Geometry check sheet. Reference: the model listing, model coordinates, mm. Face numbers are marked on the shaded views. A direction names the side the tool comes from. Coordinates: 2 decimals unless noted, no trailing zeros. Write each loop counter-clockwise with the first axis right and the second up, starting at its lowest first coordinate (ties: lowest second). Pieces come first, ordered by that corner, then holes. Notation, with made-up numbers: M 9,-25.75 L 17,-25.75 A18 cw 17,-12.75 Z; hole C 26.25,16.25 d4. An arc over 180 degrees is marked long. Write each question's results on one line, items separated by ' | '.
Autodesk Inventor part; units mm, degrees
ref_plane "YZ Plane" through (0, 0, 0) normal (1, 0, 0) x (0, 1, 0)
ref_plane "XZ Plane" through (0, 0, 0) normal (0, 1, 0) x (-1, 0, 0)
ref_plane "XY Plane" through (0, 0, 0) normal (0, 0, 1) x (1, 0, 0)
ref_plane "Work Plane1" through (0, 0, 108.3756) normal (0, 0, 1) x (1, 0, 0)
sketch "Sketch1" plane through (0, 0, 108.3756) normal (0, 0, 1) x (1, 0, 0)
  line L0 (-71.3, 18) -> (-71.3, -18)
  line L1 (-71.3, -18) -> (-211.3, -18)
  line L2 (-211.3, -18) -> (-211.3, 18)
  line L3 (-211.3, 18) -> (-71.3, 18)
  line L4 (71.3003, -18) -> (71.3003, 18)
  line L5 (71.3003, 18) -> (211.3003, 18)
  line L6 (211.3003, 18) -> (211.3003, -18)
  line L7 (211.3003, -18) -> (71.3003, -18)
  line L8 (-241.3, 22) -> (241.3, 22)
  line L9 (-241.3, -22) -> (-241.3, 22)
  line L10 (241.3, -22) -> (-241.3, -22)
  line L11 (241.3, 22) -> (241.3, -22)
  circle A0 centre (-232.5, -15.875) radius 3.5
  circle A1 centre (-232.5, 15.875) radius 3.5
  circle A2 centre (232.5, -15.875) radius 3.5
  circle A3 centre (232.5, 15.875) radius 3.5
  line L12 (-219.3, 10) -> (-219.3, -10)
  line L13 (-63.3, 10) -> (-63.3, -10)
  arc A4 (-211.3, 18) -> (-219.3, 10) centre (-211.3, 10) ccw
  arc A5 (-219.3, -10) -> (-211.3, -18) centre (-211.3, -10) ccw
  arc A6 (-63.3, 10) -> (-71.3, 18) centre (-71.3, 10) ccw
  arc A7 (-71.3, -18) -> (-63.3, -10) centre (-71.3, -10) ccw
  line L14 (-211.3, 18) -> (-71.3, 18)
  line L15 (-71.3, -18) -> (-211.3, -18)
  circle A8 centre (-215.3, 0) radius 2
  circle A9 centre (-67.3, 0) radius 2
  point P0 (0, 0)
  point P1 (-63.3, 0)
  dimension "d0" = 8
  dimension "d1" = 8
  dimension "d5" = 4
  dimension "d6" = 4
  dimension "d7" = 18
  dimension "d9" = 4
  dimension "d106" = 18
extrude "Extrusion2" add sketch "Sketch1" along normal blind 2 contours A6 L13 A7 L0 | L0 L1 L2 L3 | L2 A5 L12 A4
ref_plane "Work Plane4" through (-211.3, -18, 108.3756) normal (0, -1, 0) x (1, 0, 0)
sketch "Sketch3" plane through (-211.3, -18, 108.3756) normal (0, -1, 0) x (1, 0, 0)
  line L0 (0, 2) -> (140, 2)
  line L1 (0, 2) -> (140, 2)
  line L2 (140, 2) -> (140, 102)
  line L3 (140, 102) -> (0, 102)
  line L4 (0, 102) -> (0, 2)
  point P0 (211.3, -108.3756)
  point P1 (140, 2)
  dimension "d14" = 100
  dimension "d15" = 0
extrude "Extrusion3" add sketch "Sketch3" against normal blind 2
ref_plane "Work Plane5" through (-71.3, -18, 210.3756) normal (1, 0, 0) x (0, 0, -1)
sketch "Sketch4" plane through (-71.3, -18, 210.3756) normal (1, 0, 0) x (0, 0, -1)
  line L0 (0, 2) -> (100, 2)
  line L1 (100, 2) -> (1, 2)
  line L2 (1, 2) -> (100, 36)
  line L3 (100, 36) -> (100, 2)
  point P0 (210.3756, 18)
  dimension "d19" = 99
extrude "Side" add sketch "Sketch4" against normal blind 2
ref_plane "Work Plane6" through (-211.3, -18, 110.3756) normal (-1, 0, 0) x (0, 0, 1)
sketch "Sketch5" plane through (-211.3, -18, 110.3756) normal (-1, 0, 0) x (0, 0, 1)
  line L0 (0, 2) -> (100, 2)
  line L1 (0, 2) -> (99, 2)
  line L2 (0, 36) -> (99, 2)
  line L3 (0, 36) -> (99, 2)
  line L4 (0, 36) -> (0, 2)
  point P0 (-110.3756, 18)
extrude "Extrusion5" add sketch "Sketch5" against normal blind 2
sketch "Sketch7" plane through (0, 0, 110.3756) normal (0, 0, 1) x (1, 0, 0)
  line L0 (-209.3, -16) -> (-73.3, -16)
  line L1 (-129.3, -16) -> (-204.3, -16)
  line L2 (-134.3, 18) -> (-209.3, 18)
  line L3 (-134.3, -18) -> (-134.3, 18)
  line L4 (-209.3, 18) -> (-209.3, -16)
  line L5 (-209.3, -18) -> (-134.3, -18)
  line L6 (-209.3, -18) -> (-134.3, -18)
  line L7 (-209.3, 18) -> (-134.3, 18)
  line L8 (-134.3, 18) -> (-134.3, -18)
  line L9 (-134.3, -18) -> (-209.3, -18)
  line L10 (-209.3, -18) -> (-209.3, 18)
  point P0 (0, 0)
  point P1 (-134.3, -16)
extrude "Extrusion7" cut sketch "Sketch7" against normal through all contours L4 L2 L3 L0
sketch "Sketch14" plane through (0, 0, 108.3756) normal (0, 0, -1) x (-1, 0, 0)
  line L0 (116.3, 1.1) -> (131.8, 1.1)
  line L1 (110.85, 3.1) -> (99.75, 3.1)
  line L2 (80.95, 3.1) -> (93.65, 3.1)
  line L3 (131.8, -12.2) -> (131.8, 0.9)
  line L4 (116.3, 0.9) -> (116.3, -12.2)
  line L5 (112.15, -1.76) -> (112.15, 2.24)
  line L6 (112.15, -10.26) -> (112.15, -6.26)
  line L7 (98.05, -6.56) -> (98.05, -9.96)
  line L8 (98.05, 1.94) -> (98.05, -1.46)
  line L9 (81.3, -12.4) -> (131.3, -12.4)
  line L10 (94.1, -5.96) -> (94.1, -9.76)
  line L11 (94.1, -2.3) -> (94.1, 1.5)
  line L12 (80.5, -2.3) -> (80.5, 1.5)
  line L13 (80.5, -5.96) -> (80.5, -9.76)
  line L14 (79.5, 4.1) -> (95.1, 4.1)
  line L15 (95.1, 4.1) -> (95.1, -13.4)
  line L16 (95.1, -13.4) -> (79.5, -13.4)
  line L17 (79.5, -13.4) -> (79.5, 4.1)
  line L18 (97.05, 4.1) -> (113.15, 4.1)
  line L19 (113.15, 4.1) -> (113.15, -13.4)
  line L20 (113.15, -13.4) -> (97.05, -13.4)
  line L21 (97.05, -13.4) -> (97.05, 4.1)
  line L22 (115.3, 2.1) -> (132.8, 2.1)
  line L23 (132.8, 2.1) -> (132.8, -13.4)
  line L24 (132.8, -13.4) -> (115.3, -13.4)
  line L25 (115.3, -13.4) -> (115.3, 2.1)
  point P0 (0, 0)
  dimension "d54" = 1
  dimension "d55" = 1
  dimension "d56" = 1
  dimension "d58" = 1
  dimension "d59" = 1
  dimension "d60" = 1
  dimension "d61" = 1
  dimension "d62" = 1
  dimension "d63" = 1
  dimension "d64" = 1
  dimension "d65" = 1
  dimension "d66" = 1
extrude "Extrusion12" cut sketch "Sketch14" against normal up to surface (2 mm away)
fillet "Fillet1" radius 1.5 2 edges at (-69.3, 0, 108.3756) (-217.3, 0, 108.3756)
sketch "Sketch19" plane through (0, 0, 108.3756) normal (0, 0, -1) x (-1, 0, 0)
  circle A0 centre (67.3, 0) radius 3.5
  line L0 (79.5, 4.1) -> (95.1, 4.1)
  line L1 (95.1, 4.1) -> (95.1, -13.4)
  line L2 (95.1, -13.4) -> (79.5, -13.4)
  line L3 (79.5, -13.4) -> (79.5, 4.1)
  line L4 (132.8, -13.4) -> (115.3, -13.4)
  line L5 (115.3, -13.4) -> (115.3, 2.1)
  line L6 (115.3, 2.1) -> (132.8, 2.1)
  line L7 (132.8, 2.1) -> (132.8, -13.4)
  line L8 (97.05, -13.4) -> (97.05, 4.1)
  line L9 (97.05, 4.1) -> (113.15, 4.1)
  line L10 (113.15, 4.1) -> (113.15, -13.4)
  line L11 (113.15, -13.4) -> (97.05, -13.4)
  line L12 (209.3, 18) -> (209.3, -16)
  line L13 (209.3, -16) -> (134.3, -16)
  line L14 (134.3, -16) -> (134.3, 18)
  line L15 (71.3, 18) -> (134.3, 18)
  arc A1 (71.3, 18) -> (63.3, 10) centre (71.3, 10) ccw
  line L16 (63.3, -10) -> (63.3, 10)
  arc A2 (63.3, -10) -> (71.3, -18) centre (71.3, -10) ccw
  line L17 (211.3, -18) -> (71.3, -18)
  arc A3 (211.3, -18) -> (219.3, -10) centre (211.3, -10) ccw
  line L18 (219.3, 10) -> (219.3, -10)
  arc A4 (219.3, 10) -> (211.3, 18) centre (211.3, 10) ccw
  line L19 (209.3, 18) -> (211.3, 18)
  circle A5 centre (215.3, 0) radius 3.5
  line L20 (71.3, 21) -> (211.3, 21)
  line L21 (63.3, 10) -> (63.3, 13)
  line L22 (63.3, -10) -> (63.3, -13)
  line L23 (219.3, 10) -> (219.3, 13)
  line L24 (219.3, -10) -> (219.3, -13)
  line L25 (71.3, -21) -> (211.3, -21)
  arc A6 (211.3, -21) -> (219.3, -13) centre (211.3, -13) ccw
  arc A7 (219.3, 13) -> (211.3, 21) centre (211.3, 13) ccw
  arc A8 (71.3, 21) -> (63.3, 13) centre (71.3, 13) ccw
  arc A9 (63.3, -13) -> (71.3, -21) centre (71.3, -13) ccw
  line L26 (209.3, 18) -> (134.3, 18)
  point P0 (0, 0)
  dimension "d108" = 3
  dimension "d109" = 3
  dimension "d110" = 3
  dimension "d111" = 3
  dimension "d112" = 3
  dimension "d114" = 3
extrude "Extrusion17" add sketch "Sketch19" against normal blind 2 contours L26 L15 A1 L21 A8 L20 A7 L23 A4 L19 | L24 A6 L25 A9 L22 A2 L17 A3
sketch "Sketch20" plane through (-71.3, -18, 210.3756) normal (1, 0, 0) x (0, 0, -1)
  line L0 (100, 36) -> (1, 2)
  line L1 (1, 2) -> (1, 17)
  line L2 (102, 36) -> (100, 36)
  line L3 (1, 17) -> (100, 36)
  point P0 (210.3756, 18)
  dimension "d117" = 15
extrude "Extrusion18" add sketch "Sketch20" against normal blind 2
sketch "Sketch21" plane through (-71.3, -18, 210.3756) normal (1, 0, 0) x (0, 0, -1)
  line L0 (1, 2) -> (100, 2)
  line L1 (100, 36) -> (1, 17)
  line L2 (16, 2) -> (51, 2)
  line L3 (51, 2) -> (51, 11)
  line L4 (45, 17) -> (22, 17)
  line L5 (16, 11) -> (16, 2)
  line L6 (1, 17) -> (1, 2)
  arc A0 (22, 17) -> (16, 11) centre (22, 11) ccw
  arc A1 (51, 11) -> (45, 17) centre (45, 11) ccw
  arc A2 (16, 7) -> (21, 2) centre (21, 7) ccw
  arc A3 (46, 2) -> (51, 7) centre (46, 7) ccw
  point P0 (210.3756, 18)
  point P1 (21, 2)
  point P2 (46, 2)
  dimension "d120" = 15
  dimension "d121" = 15
  dimension "d122" = 50
  dimension "d123" = 6
  dimension "d124" = 5
  dimension "d125" = 5
extrude "Extrusion19" cut sketch "Sketch21" against normal blind 2 contours A2 L5 A0 L4 A1 L3 A3 L0
sketch "Sketch24" plane through (-211.3, -16, 108.3756) normal (0, 1, 0) x (1, 0, 0)
  circle A0 centre (129.5, -25.5) radius 1.35
  circle A1 centre (80.5, -25.5) radius 1.35
  circle A2 centre (80.5, -83.5) radius 1.35
  circle A3 centre (129.5, -83.5) radius 1.35
  circle A4 centre (129.5, -83.5) radius 3.5
  circle A5 centre (80.5, -83.5) radius 3.5
  circle A6 centre (80.5, -25.5) radius 3.5
  circle A7 centre (129.5, -25.5) radius 3.5
  point P0 (211.3, 108.3756)
  dimension "d128" = 7
  dimension "d129" = 7
  dimension "d130" = 7
  dimension "d131" = 7
extrude "Extrusion20" add sketch "Sketch24" along normal blind 2 contours A0 | A1 | A2 | A3 | A4 | A5 | A6 | A7
sketch "Sketch25" plane through (-130.8, -14, 133.8756) normal (0, 1, 0) x (1, 0, 0)
  circle A0 centre (49, 0) radius 3.5
  circle A1 centre (49, -58) radius 3.5
  circle A2 centre (0, -58) radius 3.5
  circle A3 centre (0, 0) radius 3.5
  point P0 (130.8, 133.8756)
hole "Hole1" at (-81.8, -14, 133.8756) at (-130.8, -14, 133.8756) at (-130.8, -14, 191.8756) at (-81.8, -14, 191.8756) direction (0, -1, 0) diameter 2 end through all
properties part number "RPI_HOUSING2" material "Rubber, Silicone"
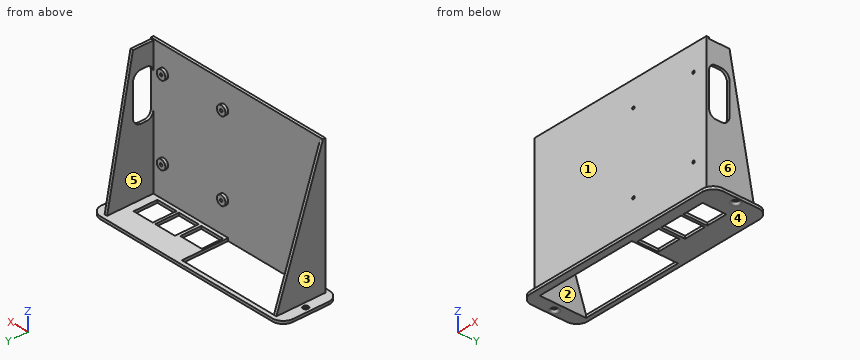
Q1. Sectioned sample at C-C on z = 174.5. Record the cut outline in (x, y), and give its area (3 significant figures).
Geometry check:
outline: M -211.3,-18 L -71.3,-18 L -71.3,-16 L -209.3,-16 L -209.3,-4.02 L -211.3,-4.02 Z; M -73.3,-1 L -71.3,-1 L -71.3,5.69 L -73.3,5.69 Z | area: 317 mm2
Q2. Depth check by flat-ended pin: P1, Ø4.5, axis at x = -67.3, y = 0, coming from the +Z side; P2, Ø2, axis at x = -129.5, z = 191, coming from the +Y side; P3, Ø10, axis at x = -153, z = 161.5, coming from the -Y side; P4, Ø8, axis at x = -158, y = -11.5, coming from the -Z side. Enter the tip coordinate at first touch or a pass-through.
Geometry check:
P1: stops at z = 110.38 | P2: stops at y = -14 | P3: stops at y = -18 | P4: passes through
Q3. Scan lines: probe 1 along X at (y, z) = (-12, 139.5); probe 2 along Z at (x, y) = (-81.8, -15.65); probe 3 along Z at (x, y) = (-81, -15). Record each from-to range of solid material in increasing order.
Geometry check:
probe 1: x = -211.3 to -209.3, -73.3 to -71.3 | probe 2: z = 108.38 to 110.38, 130.38 to 132.88, 134.88 to 137.38, 188.38 to 190.88, 192.88 to 195.38 | probe 3: z = 108.38 to 110.38, 130.47 to 133.28, 134.48 to 137.28, 188.47 to 191.28, 192.48 to 195.28
Q4. Sectioned sample at A-A on x = -144. Record the cut outline in (y, z), and give its area (3 significant figures).
Geometry check:
outline: M -21,108.38 L -16,108.38 L -16,210.38 L -18,210.38 L -18,110.38 L -21,110.38 Z; M 18,108.38 L 21,108.38 L 21,110.38 L 18,110.38 Z | area: 216 mm2
Q5. Sectioned sample at D-D on y = 15.5. Record the cut outline in (x, z), and give its area (3 significant figures).
Geometry check:
outline: M -218.9,108.38 L -209.3,108.38 L -209.3,117.66 L -211.3,117.66 L -211.3,110.38 L -218.9,110.38 Z; M -134.3,108.38 L -63.7,108.38 L -63.7,110.38 L -71.3,110.38 L -71.3,123.4 L -73.3,123.4 L -73.3,110.38 L -134.3,110.38 Z | area: 201 mm2
Q6. Sectioned sample at B-B on x = -75.5. Record the cut outline in (y, z), and give its area (3 significant figures).
Geometry check:
outline: M -21,108.38 L 21,108.38 L 21,110.38 L -16,110.38 L -16,210.38 L -18,210.38 L -18,110.38 L -21,110.38 Z | area: 284 mm2
Q7. Access from +Z, -Z, +X, -X, +Y, -Y to the whole of each face (thin tool, end or side, straight path). Record for the marked faces 4, 5 and 6.
Geometry check:
face 4: -Z, +X, -X, +Y, -Y | face 5: +Z, +Y | face 6: +Z, +X, +Y, -Y
Q8. Mould release check, pull along X, two halves, no side actions. Record for the marked faces 1, 2 and 3: pulls with the +X half, pulls with the -X half, needs draft (parallel to the pull), parting line crosses it, or undercut.
Geometry check:
face 1: needs draft | face 2: undercut | face 3: pulls with the -X half
